```python
from build123d import *

# Parameters (mm, degrees)
EXTRUDE_1_DEPTH      = 164.95
EXTRUDE_1_DEPTH_BACK = 164.95
SKETCH_1_R           = 4
SKETCH_2_R           = 1.5
EXTRUDE_2_DEPTH      = 5
FILLET_1_R           = 0.5


with BuildPart() as part:
    # Эскиз1 → Выдавливание1 (new, two sides: drawn at the far end of the back side and taken through both)
    with BuildSketch(Plane(origin=(0, 0, 0), x_dir=(-1, 0, 0), z_dir=(0, 1, 0)).offset(-EXTRUDE_1_DEPTH_BACK)):
        with Locations(Location((0, 0, 0), (0, 0, 90))):
            Circle(SKETCH_1_R)
    extrude(amount=EXTRUDE_1_DEPTH + EXTRUDE_1_DEPTH_BACK)

    # Эскиз2 → Выдавливание2 (cut)
    with BuildSketch(Plane(origin=(0, 164.95, 0), x_dir=(-1, 0, 0), z_dir=(0, 1, 0))):
        with Locations(Location((0, 0, 0), (0, 0, 90))):
            Circle(SKETCH_2_R)
    extrude_2 = extrude(amount=-EXTRUDE_2_DEPTH, mode=Mode.SUBTRACT)

    # Зеркальное отражение1: Выдавливание2 across plane
    add(extrude_2.mirror(Plane.ZX), mode=Mode.SUBTRACT)

    # Сопряжение1
    fillet_1_edges = [part.edges().sort_by_distance(p)[0] for p in [
        (0, -164.95, -4),
        (0, 164.95, -4),
    ]]
    fillet(fillet_1_edges, radius=FILLET_1_R)


solid = part.part
```
Geometry: final body of the model. Coordinates: model frame, mm. Give positions to 0.01 mm unless a question says otherwise; leave off trailing zeros. Loops run counter-clockwise (first coordinate to the right, second up) from the corner with the lowest first, then second, coordinate; pieces in that order, holes last. Notation, with made-up numbers: (88, 37.5) -> (139, 37.5) arc R17 ccw to (139, 58.5) -> close; hole circle Ø7 at (45, 16). An arc over 180 degrees is marked (long way). Return JSON: item names as keys, results as strings.
Item 1: Section A-A, the plane y = -72.5. Output: boundary loops of the cut face in (x, z).
Filled in:
{"outline": "circle Ø8 at (0, 0)"}
Item 2: Pin query (flat end, axial travel): P1, Ø2.5, axis at x = 0, z = 0, coming from the +Y side; P2, Ø1.5, axis at x = -2.5, y = -71, coming from the +Z side; P3, Ø2.5, axis at x = 0, z = 0, coming from the -Y side. Return the tip coordinate at first contact, or that it passes through.
Filled in:
{"P1": "y = 159.95", "P2": "z = 3.6", "P3": "y = -159.95"}
Item 3: Line query: line 1 (X direction, y = -162.25, z = 0); line 2 (Z direction, x = -2, y = -115). Output: solid intervals per line, ascending.
Filled in:
{"line 1": "-4 to -1.5, 1.5 to 4", "line 2": "-3.46 to 3.46"}
